Here's how the part is built. I have some questions about the finished solid (model axes, mm). Round coordinates to 2 decimals unless told otherwise and drop trailing zeros. Answer as a JSON object with one key per item and string values.
from build123d import *

# Parameters (mm, degrees)
F0_R     = 101.6
F0_R_2   = 3.175
F0_R_3   = 4.7625
F0_R_4   = 28.575
F1_DEPTH = 2.38125
F2_W     = 23.27275
F2_H     = 3.175
F4_SIZE  = 0.25399


# Not quite as in the source:
# - a fillet or chamfer is up to 0.001 mm smaller than in the source, because OpenCascade refuses the exact size


with BuildPart() as f1:
    # F0 (on Right) → F1 (new body, symmetric)
    with BuildSketch(Plane.YZ):
        Circle(F0_R)
        with Locations((-62.4282468049, -65.9764627324)):
            Circle(F0_R_2, mode=Mode.SUBTRACT)
        with Locations((-66.9177945797, -53.478147823)):
            Circle(F0_R_2, mode=Mode.SUBTRACT)
        with Locations((-12.5679149295, -77.0653458753)):
            Circle(F0_R_2, mode=Mode.SUBTRACT)
        with Locations((0, -81.3562)):
            Circle(F0_R_2, mode=Mode.SUBTRACT)
        with Locations((-24.7782971774, -71.843231346)):
            Circle(F0_R_2, mode=Mode.SUBTRACT)
        with Locations((-70.4565359554, -40.6781)):
            Circle(F0_R_2, mode=Mode.SUBTRACT)
        with Locations((-73.0245047442, -27.6485393361)):
            Circle(F0_R_2, mode=Mode.SUBTRACT)
        with Locations((-74.6072120243, -14.4629808549)):
            Circle(F0_R_2, mode=Mode.SUBTRACT)
        with Locations((-28.0633003783, -28.0633003783)):
            Circle(F0_R_3, mode=Mode.SUBTRACT)
        with Locations((0, -39.6875)):
            Circle(F0_R_3, mode=Mode.SUBTRACT)
        with Locations((-39.6875, 0)):
            Circle(F0_R_3, mode=Mode.SUBTRACT)
        Circle(F0_R_4, mode=Mode.SUBTRACT)
        with Locations((12.8545372722, -84.6915839827)):
            Circle(F0_R_2, mode=Mode.SUBTRACT)
        with Locations((25.9231693756, -87.052679013)):
            Circle(F0_R_2, mode=Mode.SUBTRACT)
        with Locations((49.8289148469, -57.3802504911)):
            Circle(F0_R_2, mode=Mode.SUBTRACT)
        with Locations((28.0633003783, -28.0633003783)):
            Circle(F0_R_3, mode=Mode.SUBTRACT)
        with Locations((39.6875, 0)):
            Circle(F0_R_3, mode=Mode.SUBTRACT)
        with Locations((60.4565898147, -49.4168065392)):
            Circle(F0_R_2, mode=Mode.SUBTRACT)
        with Locations((70.4565359554, -40.6781)):
            Circle(F0_R_2, mode=Mode.SUBTRACT)
        with Locations((79.7723318519, -31.2134361597)):
            Circle(F0_R_2, mode=Mode.SUBTRACT)
        with Locations((88.3514161805, -21.0762162806)):
            Circle(F0_R_2, mode=Mode.SUBTRACT)
        with Locations((-88.3514161805, 21.0762162806)):
            Circle(F0_R_2, mode=Mode.SUBTRACT)
        with Locations((-79.7723318519, 31.2134361597)):
            Circle(F0_R_2, mode=Mode.SUBTRACT)
        with Locations((-70.4565359554, 40.6781)):
            Circle(F0_R_2, mode=Mode.SUBTRACT)
        with Locations((-60.4565898147, 49.4168065392)):
            Circle(F0_R_2, mode=Mode.SUBTRACT)
        with Locations((-28.0633003783, 28.0633003783)):
            Circle(F0_R_3, mode=Mode.SUBTRACT)
        with Locations((0, 39.6875)):
            Circle(F0_R_3, mode=Mode.SUBTRACT)
        with Locations((-49.8289148469, 57.3802504911)):
            Circle(F0_R_2, mode=Mode.SUBTRACT)
        with Locations((-25.9231693756, 87.052679013)):
            Circle(F0_R_2, mode=Mode.SUBTRACT)
        with Locations((-12.8545372722, 84.6915839827)):
            Circle(F0_R_2, mode=Mode.SUBTRACT)
        with Locations((0, 81.3562)):
            Circle(F0_R_2, mode=Mode.SUBTRACT)
        with Locations((28.0633003783, 28.0633003783)):
            Circle(F0_R_3, mode=Mode.SUBTRACT)
        with Locations((74.6072120243, 14.4629808549)):
            Circle(F0_R_2, mode=Mode.SUBTRACT)
        with Locations((73.0245047442, 27.6485393361)):
            Circle(F0_R_2, mode=Mode.SUBTRACT)
        with Locations((70.4565359554, 40.6781)):
            Circle(F0_R_2, mode=Mode.SUBTRACT)
        with Locations((24.7782971774, 71.843231346)):
            Circle(F0_R_2, mode=Mode.SUBTRACT)
        with Locations((12.5679149295, 77.0653458753)):
            Circle(F0_R_2, mode=Mode.SUBTRACT)
        with Locations((66.9177945797, 53.478147823)):
            Circle(F0_R_2, mode=Mode.SUBTRACT)
        with Locations((62.4282468049, 65.9764627324)):
            Circle(F0_R_2, mode=Mode.SUBTRACT)
    extrude(amount=F1_DEPTH, both=True)

    # F2 (on Front) → F3 (revolve, cut)
    with BuildSketch(Plane.XZ):
        with Locations((-13.763625, 61.9125)):
            Rectangle(F2_W, F2_H)
        with Locations((13.763625, 61.9125)):
            Rectangle(F2_W, F2_H)
    revolve(axis=Axis((-12.7, 0, 0), (-1, 0, 0)), mode=Mode.SUBTRACT)

    # F4 (size 0.254 in the source; OpenCascade refuses exactly that, so slightly less here)
    f4_edges = [f1.edges().sort_by_distance(p)[0] for p in [
        (-2.38125, -101.6, 0),
        (-2.38125, -65.603247, -65.976463),
        (-2.38125, -70.092795, -53.478148),
        (-2.38125, -27.953297, -71.843231),
        (-2.38125, -3.175, -81.3562),
        (-2.38125, -15.742915, -77.065346),
        (-2.38125, -73.631536, -40.6781),
        (-2.38125, -76.199505, -27.648539),
        (-2.38125, -77.782212, -14.462981),
        (-2.38125, 9.679537, -84.691584),
        (-2.38125, 22.748169, -87.052679),
        (-2.38125, 46.653915, -57.38025),
        (-2.38125, 57.28159, -49.416807),
        (-2.38125, 67.281536, -40.6781),
        (-2.38125, 76.597332, -31.213436),
        (-2.38125, 85.176416, -21.076216),
        (-2.38125, -91.526416, 21.076216),
        (-2.38125, -82.947332, 31.213436),
        (-2.38125, -73.631536, 40.6781),
        (-2.38125, 0, -63.5),
        (-2.38125, -63.63159, 49.416807),
        (-2.38125, -53.003915, 57.38025),
        (-2.38125, -29.098169, 87.052679),
        (-2.38125, -16.029537, 84.691584),
        (-2.38125, -3.175, 81.3562),
        (-2.38125, 71.432212, 14.462981),
        (-2.38125, 69.849505, 27.648539),
        (-2.38125, 67.281536, 40.6781),
        (-2.38125, 9.392915, 77.065346),
        (-2.38125, 21.603297, 71.843231),
        (-2.38125, 63.742795, 53.478148),
        (-2.38125, 59.253247, 65.976463),
        (-2.38125, 0, -60.325),
        (-2.38125, -32.8258, -28.0633),
        (-2.38125, -4.7625, -39.6875),
        (-2.38125, 23.3008, -28.0633),
        (-2.38125, -44.45, 0),
        (-2.38125, -28.575, 0),
        (-2.38125, -32.8258, 28.0633),
        (-2.38125, -4.7625, 39.6875),
        (-2.38125, 34.925, 0),
        (-2.38125, 23.3008, 28.0633),
        (2.38125, 0, -60.325),
        (2.38125, -32.8258, -28.0633),
        (2.38125, -4.7625, -39.6875),
        (2.38125, 23.3008, -28.0633),
        (2.38125, -44.45, 0),
        (2.38125, -28.575, 0),
        (2.38125, -32.8258, 28.0633),
        (2.38125, -4.7625, 39.6875),
        (2.38125, 34.925, 0),
        (2.38125, 23.3008, 28.0633),
        (2.38125, -101.6, 0),
        (2.38125, -65.603247, -65.976463),
        (2.38125, -70.092795, -53.478148),
        (2.38125, -27.953297, -71.843231),
        (2.38125, -3.175, -81.3562),
        (2.38125, -15.742915, -77.065346),
        (2.38125, -73.631536, -40.6781),
        (2.38125, -76.199505, -27.648539),
        (2.38125, -77.782212, -14.462981),
        (2.38125, 9.679537, -84.691584),
        (2.38125, 22.748169, -87.052679),
        (2.38125, 46.653915, -57.38025),
        (2.38125, 57.28159, -49.416807),
        (2.38125, 67.281536, -40.6781),
        (2.38125, 76.597332, -31.213436),
        (2.38125, 85.176416, -21.076216),
        (2.38125, -91.526416, 21.076216),
        (2.38125, -82.947332, 31.213436),
        (2.38125, -73.631536, 40.6781),
        (2.38125, 0, -63.5),
        (2.38125, -63.63159, 49.416807),
        (2.38125, -53.003915, 57.38025),
        (2.38125, -29.098169, 87.052679),
        (2.38125, -16.029537, 84.691584),
        (2.38125, -3.175, 81.3562),
        (2.38125, 71.432212, 14.462981),
        (2.38125, 69.849505, 27.648539),
        (2.38125, 67.281536, 40.6781),
        (2.38125, 9.392915, 77.065346),
        (2.38125, 21.603297, 71.843231),
        (2.38125, 63.742795, 53.478148),
        (2.38125, 59.253247, 65.976463),
    ]]
    chamfer(f4_edges, length=F4_SIZE)


solid = f1.part
Item 1: I want a section at A-A, the plane z = 0. State how many separate pieces and enclosed holes the cut face has, then the cut area to 3 significant figures.
Resolved:
{"separate pieces": "4", "enclosed holes": "0", "area": "601 mm²"}
Item 2: I'm going to push flat-ended pins straight in: pin 1 Ø2 at (x, z) = (-1, 8) entering from +Y; pin 2 Ø1 at (x, y) = (-1.5, -76.5) entering from +Z. Where does each tip first touch, or does it pass through?
Resolved:
{"pin 1": "y = 101.36", "pin 2": "z = 67.43"}
Item 3: Please list where these lines run through material, in increasing order: probe 1 along Z at (x, y) = (-1.15, 0) (3 decimals); probe 2 along Z at (x, y) = (-0.2, -62); probe 3 along Z at (x, y) = (-0.2, -59.5). Write a range as from..to.
Resolved:
{"probe 1": "-101.6..-84.531, -78.181..-44.45, -34.925..-28.575, 28.575..34.925, 44.45..78.181, 84.531..101.6", "probe 2": "-80.49..-69.12, -62.83..46.64, 52.19..80.49", "probe 3": "-82.35..-67.2, -64.75..46.39, 52.44..82.35"}
